Read the model definition and answer for the solid it produces. Units are mm, in the model's axes. A direction names the side the tool comes from. Round coordinates to 2 decimals unless told otherwise and drop trailing zeros. Loops run counter-clockwise (first coordinate to the right, second up) from the corner with the lowest first, then second, coordinate; pieces in that order, holes last. Notation, with made-up numbers: (23.5, -27.75) -> (47.5, -27.75) arc R19 cw to (47.5, -19.75) -> close; hole circle Ø3 at (68, 24). An arc over 180 degrees is marked (long way). Put each result on its own line as item: value.
from build123d import *

# Parameters (mm, degrees)
SKETCH1_W                                 = 85
SKETCH1_H                                 = 60
BOSS_EXTRUDE1_DEPTH                       = 100
CUT_EXTRUDE1_START                        = 5
SKETCH2_W                                 = 35
SKETCH2_H                                 = 55
CUT_EXTRUDE1_DEPTH                        = 95
SKETCH3_W                                 = 85
SKETCH3_H                                 = 5
BOSS_EXTRUDE2_DEPTH                       = 70
BOSS_EXTRUDE3_DEPTH                       = 10
SKETCH5_W                                 = 20
SKETCH5_H                                 = 2.5
CUT_EXTRUDE2_DEPTH                        = 7.5
SKETCH6_W                                 = 35
SKETCH6_H                                 = 12
CUT_EXTRUDE4_DEPTH                        = 57.5
CUT_EXTRUDE6_REACH                        = 186.73
SKETCH7_R                                 = 4
SKETCH9_W                                 = 85
SKETCH9_H                                 = 50
BOSS_EXTRUDE4_DEPTH                       = 5
SKETCH13_W                                = 8
SKETCH13_H                                = 7
CUT_EXTRUDE8_BUTTON_HOLES_DEPTH           = 169.374582405
SKETCH14_W                                = 28
SKETCH14_H                                = 28
BOSS_EXTRUDE5_OLED_MOUNT_DEPTH            = 10
BOSS_EXTRUDE6_OLED_MOUNT_DEPTH            = 1
BOSS_EXTRUDE7_START                       = -2.5
BOSS_EXTRUDE7_OLED_MOUNT_DEPTH            = 1
CHAMFER2_OLED_MOUNT_SIZE                  = 10
CUT_EXTRUDE7_START                        = -40.5
CUT_EXTRUDE7_OLED_CABLE_HOLE_DEPTH        = 4
CUT_EXTRUDE7_ROOF_CUTOUT_DEPTH            = 172.245437895
SKETCH18_W                                = 4
SKETCH18_H                                = 8
CUT_EXTRUDE9_OLED_CABLE_DEPTH             = 153.213665615
CHAMFER6_OLED_CABLE_HOLE_SIZE             = 2.5
CHAMFER6_OLED_CABLE_HOLE_SIZE2            = 4.330127019
SKETCH45_R                                = 1.5
CUT_EXTRUDE7_ROOF_HOLES_DEPTH             = 15
SKETCH20_W                                = 10
SKETCH20_H                                = 10
CUT_EXTRUDE10_SOLENOID_WIRE_HOLE_DEPTH    = 169.374582405
SKETCH21_W                                = 5
SKETCH21_H                                = 32
BOSS_EXTRUDE9_SOLENOID_SIDE_SUPPORT_DEPTH = 5
CHAMFER3_THUMB_SIZE                       = 2.5
CHAMFER5_THUMB_SIZE                       = 4.5
CHAMFER5_THUMB_SIZE2                      = 7.794228634
CHAMFER5_THUMB_PART_2_SIZE                = 4.5
CHAMFER5_THUMB_PART_2_SIZE2               = 7.794228634
CHAMFER5_THUMB_PART_3_SIZE                = 4.5
CHAMFER5_THUMB_PART_3_SIZE2               = 7.794228634
BOSS_EXTRUDE5_GUIDE_DEPTH                 = 180
SKETCH42_W                                = 10
SKETCH42_H                                = 70
BOSS_EXTRUDE8_DEPTH                       = 10
CHAMFER5_SIZE                             = 10
CHAMFER5_SIZE_2                           = 71.153697224


# Some blends are built 0.0001 mm under size
with BuildPart() as part:
    # Sketch1 → Boss-Extrude1 (new body)
    with BuildSketch(Plane(origin=(0, 0, 0), x_dir=(1, 0, 0), z_dir=(0, 1, 0))):
        with Locations((42.5, 30)):
            Rectangle(SKETCH1_W, SKETCH1_H)
    extrude(amount=BOSS_EXTRUDE1_DEPTH)

    # Sketch2 → Cut-Extrude1 (cut)
    with BuildSketch(Plane(origin=(0, 0, 0), x_dir=(1, 0, 0), z_dir=(0, 1, 0)).offset(CUT_EXTRUDE1_START)):
        with Locations((20, 30)):
            Rectangle(SKETCH2_W, SKETCH2_H)
        with Locations((65, 30)):
            Rectangle(SKETCH2_W, SKETCH2_H)
    extrude(amount=CUT_EXTRUDE1_DEPTH, mode=Mode.SUBTRACT)

    # Sketch3 → Boss-Extrude2 (add)
    with BuildSketch(Plane.XY):
        with Locations((42.5, 2.5)):
            Rectangle(SKETCH3_W, SKETCH3_H)
    extrude(amount=BOSS_EXTRUDE2_DEPTH)

    # Sketch4 → Boss-Extrude3 (add)
    with BuildSketch(Plane(origin=(0, 5, 0), x_dir=(1, 0, 0), z_dir=(0, 1, 0))):
        Polygon((85, 0), (82.5, 0), (82.5, -67.5), (47.5, -67.5), (47.5, 0), (37.5, 0), (37.5, -67.5), (2.5, -67.5), (2.5, 0), (0, 0), (0, -70), (85, -70), align=None)
    extrude(amount=BOSS_EXTRUDE3_DEPTH)

    # Sketch5 → Cut-Extrude2 (cut)
    with BuildSketch(Plane(origin=(0, 15, 0), x_dir=(1, 0, 0), z_dir=(0, 1, 0))):
        with Locations((20, -68.75)):
            Rectangle(SKETCH5_W, SKETCH5_H)
        with Locations((65, -68.75)):
            Rectangle(SKETCH5_W, SKETCH5_H)
    extrude(amount=-CUT_EXTRUDE2_DEPTH, mode=Mode.SUBTRACT)

    # Sketch6 → Cut-Extrude4 (cut)
    with BuildSketch(Plane.XY):
        with Locations((20, 11)):
            Rectangle(SKETCH6_W, SKETCH6_H)
        with Locations((65, 11)):
            Rectangle(SKETCH6_W, SKETCH6_H)
    extrude(amount=-CUT_EXTRUDE4_DEPTH, mode=Mode.SUBTRACT)

    # Sketch7 → Cut-Extrude6 (cut, up to next)
    with BuildSketch(Plane(origin=(0, 0, -60), x_dir=(-1, 0, 0), z_dir=(0, 0, -1)), mode=Mode.PRIVATE) as cut_extrude6_sk1:
        with Locations((-20, 11.5)):
            Circle(SKETCH7_R)
    cut_extrude6_tool1 = extrude(cut_extrude6_sk1.sketch, amount=-CUT_EXTRUDE6_REACH, mode=Mode.PRIVATE) & part.part
    # Sketch7 → Cut-Extrude6 (cut, up to next)
    with BuildSketch(Plane(origin=(0, 0, -60), x_dir=(-1, 0, 0), z_dir=(0, 0, -1)), mode=Mode.PRIVATE) as cut_extrude6_sk2:
        with Locations((-65, 11.5)):
            Circle(SKETCH7_R)
    cut_extrude6_tool2 = extrude(cut_extrude6_sk2.sketch, amount=-CUT_EXTRUDE6_REACH, mode=Mode.PRIVATE) & part.part
    add(cut_extrude6_tool1.solids().sort_by_distance((20, 11.5, -60))[0], mode=Mode.SUBTRACT)
    add(cut_extrude6_tool2.solids().sort_by_distance((65, 11.5, -60))[0], mode=Mode.SUBTRACT)

    # Sketch9 → Boss-Extrude4 (add)
    with BuildSketch(Plane(origin=(0, 0, 0), x_dir=(1, 0, 0), z_dir=(0, 1, 0))):
        with Locations((42.5, 85)):
            Rectangle(SKETCH9_W, SKETCH9_H)
    extrude(amount=BOSS_EXTRUDE4_DEPTH)

    # Sketch13 → Cut-Extrude8 (Button Holes) (cut, through all)
    with BuildSketch(Plane(origin=(0, 5, 0), x_dir=(1, 0, 0), z_dir=(0, 1, 0))):
        with Locations((20, -61)):
            Rectangle(SKETCH13_W, SKETCH13_H)
        with Locations((65, -61)):
            Rectangle(SKETCH13_W, SKETCH13_H)
    extrude(amount=-CUT_EXTRUDE8_BUTTON_HOLES_DEPTH, mode=Mode.SUBTRACT)

    # Sketch14 → Boss-Extrude5 (OLED Mount) (add)
    with BuildSketch(Plane.XY):
        Polygon((18.5, 93.172660782), (18.5, 52), (66.5, 52), (66.5, 93.172660782), (66.5, 100), (18.5, 100), align=None)
        with Locations((42.5, 76)):
            Rectangle(SKETCH14_W, SKETCH14_H, mode=Mode.SUBTRACT)
    extrude(amount=BOSS_EXTRUDE5_OLED_MOUNT_DEPTH)

    # Sketch40 → Boss-Extrude6 (OLED Mount) (add)
    with BuildSketch(Plane.XY.offset(10)):
        Polygon((28.5, 62), (36.5, 62), (28.5, 66), align=None)
        Polygon((56.5, 62), (48.5, 62), (56.5, 66), align=None)
    extrude(amount=-BOSS_EXTRUDE6_OLED_MOUNT_DEPTH)

    # Sketch40<2> → Boss-Extrude7 (OLED Mount) (add)
    with BuildSketch(Plane.XY.offset(10).offset(BOSS_EXTRUDE7_START)):
        Polygon((28.5, 62), (36.5, 62), (28.5, 66), align=None)
        Polygon((56.5, 62), (48.5, 62), (56.5, 66), align=None)
    extrude(amount=-BOSS_EXTRUDE7_OLED_MOUNT_DEPTH)

    # Chamfer2 (OLED Mount)
    chamfer2_oled_mount_edges = [part.edges().sort_by_distance(p)[0] for p in [
        (42.5, 52, 10),
        (66.5, 76, 10),
        (42.5, 100, 10),
        (18.5, 76, 10),
    ]]
    chamfer(chamfer2_oled_mount_edges, length=CHAMFER2_OLED_MOUNT_SIZE - 0.0001)  # a hair under: the kernel refuses the full size

    # Sketch44 → Cut-Extrude7 (OLED Cable Hole) (cut)
    with BuildSketch(Plane(origin=(85, 0, 0), x_dir=(0, 0, -1), z_dir=(1, 0, 0)).offset(CUT_EXTRUDE7_START)):
        Polygon((0, 62), (0, 72), (10.5, 62), align=None)
    extrude(amount=-CUT_EXTRUDE7_OLED_CABLE_HOLE_DEPTH, mode=Mode.SUBTRACT)

    # Sketch41 → Cut-Extrude7 (Roof Cutout) (cut, through all)
    with BuildSketch(Plane.XY):
        Polygon((18.5, 100), (28.5, 90), (56.5, 90), (66.5, 100), align=None)
    extrude(amount=CUT_EXTRUDE7_ROOF_CUTOUT_DEPTH, mode=Mode.SUBTRACT)

    # Sketch18 → Cut-Extrude9 (OLED Cable) (cut, through all)
    with BuildSketch(Plane(origin=(0, 62, 0), x_dir=(1, 0, 0), z_dir=(0, 1, 0))):
        with Locations((42.5, 6.5)):
            Rectangle(SKETCH18_W, SKETCH18_H)
    extrude(amount=-CUT_EXTRUDE9_OLED_CABLE_DEPTH, mode=Mode.SUBTRACT)

    # Chamfer6 (OLED Cable Hole)
    chamfer6_oled_cable_hole_edges = [part.edges().sort_by_distance(p)[0] for p in [
        (42.5, 62, -2.5),
    ]]
    chamfer6_oled_cable_hole_side = [part.faces().sort_by_distance(p)[0] for p in [
        (42.5, 62, 4.354651163),
    ]]
    chamfer(chamfer6_oled_cable_hole_edges, length=CHAMFER6_OLED_CABLE_HOLE_SIZE, length2=CHAMFER6_OLED_CABLE_HOLE_SIZE2, reference=chamfer6_oled_cable_hole_side[0])

    # Sketch45 → Cut-Extrude7 (Roof Holes) (cut)
    with BuildSketch(Plane(origin=(0, 100, 0), x_dir=(1, 0, 0), z_dir=(0, 1, 0))):
        with Locations(Location((25.5, -3, 0), (0, 0, 270))):
            Circle(SKETCH45_R)
        with Locations((59.5, -3)):
            Circle(SKETCH45_R)
    extrude(amount=-CUT_EXTRUDE7_ROOF_HOLES_DEPTH, mode=Mode.SUBTRACT)

    # Sketch20 → Cut-Extrude10 (Solenoid Wire Hole) (cut, through all)
    with BuildSketch(Plane(origin=(0, 5, 0), x_dir=(1, 0, 0), z_dir=(0, 1, 0))):
        with Locations((65, 65)):
            Rectangle(SKETCH20_W, SKETCH20_H)
        with Locations((20, 65)):
            Rectangle(SKETCH20_W, SKETCH20_H)
    extrude(amount=-CUT_EXTRUDE10_SOLENOID_WIRE_HOLE_DEPTH, mode=Mode.SUBTRACT)

    # Sketch21 → Boss-Extrude9 (Solenoid Side Support) (add)
    with BuildSketch(Plane(origin=(0, 5, 0), x_dir=(1, 0, 0), z_dir=(0, 1, 0))):
        with Locations((75, 76)):
            Rectangle(SKETCH21_W, SKETCH21_H)
        with Locations((55, 76)):
            Rectangle(SKETCH21_W, SKETCH21_H)
        with Locations((30, 76)):
            Rectangle(SKETCH21_W, SKETCH21_H)
        with Locations((10, 76)):
            Rectangle(SKETCH21_W, SKETCH21_H)
    extrude(amount=BOSS_EXTRUDE9_SOLENOID_SIDE_SUPPORT_DEPTH)

    # Chamfer3 (Thumb)
    chamfer3_thumb_edges = [part.edges().sort_by_distance(p)[0] for p in [
        (20, 7.5, 67.5),
        (65, 7.5, 67.5),
    ]]
    chamfer(chamfer3_thumb_edges, length=CHAMFER3_THUMB_SIZE - 0.0001)  # a hair under: the kernel refuses the full size

    # Chamfer5 (Thumb)
    chamfer5_thumb_edges = [part.edges().sort_by_distance(p)[0] for p in [
        (75, 15, 68.75),
    ]]
    chamfer5_thumb_side = [part.faces().sort_by_distance(p)[0] for p in [
        (83.266129032, 15, 38.266129032),
    ]]
    chamfer(chamfer5_thumb_edges, length=CHAMFER5_THUMB_SIZE, length2=CHAMFER5_THUMB_SIZE2, reference=chamfer5_thumb_side[0])

    # Chamfer5 (Thumb) part 2
    chamfer5_thumb_part_2_edges = [part.edges().sort_by_distance(p)[0] for p in [
        (55, 15, 68.75),
        (30, 15, 68.75),
    ]]
    chamfer5_thumb_part_2_side = [part.faces().sort_by_distance(p)[0] for p in [
        (42.5, 15, 36.716101695),
    ]]
    chamfer(chamfer5_thumb_part_2_edges, length=CHAMFER5_THUMB_PART_2_SIZE, length2=CHAMFER5_THUMB_PART_2_SIZE2, reference=chamfer5_thumb_part_2_side[0])

    # Chamfer5 (Thumb) part 3
    chamfer5_thumb_part_3_edges = [part.edges().sort_by_distance(p)[0] for p in [
        (10, 15, 68.75),
    ]]
    chamfer5_thumb_part_3_side = [part.faces().sort_by_distance(p)[0] for p in [
        (1.733870968, 15, 38.266129032),
    ]]
    chamfer(chamfer5_thumb_part_3_edges, length=CHAMFER5_THUMB_PART_3_SIZE, length2=CHAMFER5_THUMB_PART_3_SIZE2, reference=chamfer5_thumb_part_3_side[0])

    # Sketch37 → Boss-Extrude5 (Guide) (add, through all)
    with BuildSketch(Plane.XY.offset(70)):
        Polygon((85, 0), (88, 0), (85, 3), align=None)
        Polygon((0, 0), (-3, 0), (0, 3), align=None)
    extrude(amount=-BOSS_EXTRUDE5_GUIDE_DEPTH)

    # Sketch42 → Boss-Extrude8 (add)
    with BuildSketch(Plane(origin=(0, 15, 0), x_dir=(1, 0, 0), z_dir=(0, 1, 0))):
        with Locations((42.5, -35)):
            Rectangle(SKETCH42_W, SKETCH42_H)
    extrude(amount=BOSS_EXTRUDE8_DEPTH)

    # Chamfer5
    # the kernel refuses this chamfer: 71.153697224, 10 mm, written as the material it takes off along each edge
    with BuildSketch(Plane(origin=(232.433017826, 25, 70), x_dir=(0, -0.965159882585439, 0.2616608511941778), z_dir=(-1, 0, 0))) as chamfer5_piece_1_section:
        Polygon((CHAMFER5_SIZE * 0.965159882585, -CHAMFER5_SIZE * 0.261660851194), (-CHAMFER5_SIZE_2 * 0.261660851194, -CHAMFER5_SIZE_2 * 0.965159882583), (0, 0), align=None)
    chamfer5_piece_1 = extrude(amount=379.866035651, mode=Mode.PRIVATE)
    chamfer5_piece_1 = split(chamfer5_piece_1, bisect_by=Plane(origin=(42.5, 22.433038023, 0), z_dir=(0, 0, 1)), keep=Keep.TOP, mode=Mode.PRIVATE)
    add(chamfer5_piece_1, mode=Mode.SUBTRACT)


solid = part.part
Item 1: For a pull along Z with two mould halves and no side action, classify faces 1 (the flat face through (10, 7, -92)), 2 (the flat face through (16, 3, 61)), 3 (the flat face through (27.5, 7, -76)) as pulls with the +Z half, pulls with the -Z half, needs draft (parallel to the pull), parting line crosses it, or undercut.
Derived:
face 1: pulls with the -Z half
face 2: undercut
face 3: needs draft
Item 2: Which of the six approach directions +Z, -Z, +X, -X, +Y, -Y give full straight-line access (tool end or side, diameter ignored) to faces 4 (the flat face through (24.5, 94, 4.9)), 5 (the flat face through (12.5, 7, -76)), 6 (the flat face through (54, 63, 6.5)), 7 (the flat face through (77.5, 7, -76)), 8 (the flat face through (70, 3, -65))?
Derived:
face 4: +Z, +Y
face 5: -Z, +Y
face 6: +Y
face 7: -Z, +X, +Y
face 8: +Y, -Y
Item 3: The part is cut by section D-D (z = -25). Determine the outline of the cut face in (x, y), then the cut area to 3 significant figures.
Derived:
outline: (-3, 0) -> (88, 0) -> (85, 3) -> (85, 100) -> (82.5, 100) -> (82.5, 5) -> (47.5, 5) -> (47.5, 100) -> (37.5, 100) -> (37.5, 5) -> (2.5, 5) -> (2.5, 100) -> (0, 100) -> (0, 3) -> close
area: 1,860 mm^2
Item 4: Find the intervals of material crossed by line 1 along X through (y, z) = (67, -25.5); line 2 along Y through (x, z) = (65, -58.3); line 3 along Z through (x, y) = (59, 92), in increasing order.
Derived:
line 1: x = 0 to 2.5, 37.5 to 47.5, 82.5 to 85
line 2: y = 0 to 7.5, 15.5 to 100
line 3: z = -60 to -57.5, -2.5 to 1.59, 4.41 to 7.5
Item 5: The part is cut by section A-A (z = -66). State how many separate pieces and enclosed holes the cut face has, then the cut area to 3 significant figures.
Derived:
separate pieces: 3
enclosed holes: 0
area: 434 mm^2
Item 6: Flat-ended cylindrical pins translate along their axes: pin 1 Ø12 at (x, z) = (18, -10) entering from -Y; pin 2 Ø1 at (x, z) = (42, 50.5) entering from +Y; pin 3 Ø4 at (y, z) = (8, -75) entering from -X; pin 4 Ø3 at (y, z) = (29.5, -6.5) entering from +X. Find the tip coordinate at first contact, or state that the pin passes through.
Derived:
pin 1: stops at y = 0
pin 2: stops at y = 17.81
pin 3: stops at x = 7.5
pin 4: stops at x = 85
